```python
from build123d import *

# Parameters (mm, degrees)
BASEHEAD_DEPTH = 10
SKETCH4_W      = 0.8
SKETCH4_H      = 12.088457268


# Read off the part's stored shape, not the designer's step: HeadChamfer
with BuildPart() as part:
    # Sketch1 → BaseHead (new body)
    with BuildSketch(Plane(origin=(0, 0, 0), x_dir=(0, 0, -1), z_dir=(1, 0, 0))):
        Polygon((13.5, 7.794228634), (13.5, -7.794228634), (0, -15.588457268), (-13.5, -7.794228634), (-13.5, 7.794228634), (0, 15.588457268), align=None)
    extrude(amount=BASEHEAD_DEPTH)

    # HeadChamfer outline → HeadChamfer (revolve, cut)
    with BuildSketch(Plane.YX):
        Polygon((15.58845727, 1.205771367), (13.499999851, -8.6e-08), (15.58845727, -8.6e-08), align=None)
    revolve(axis=Axis((0, 0, 0), (1, 0, 0)), mode=Mode.SUBTRACT)

    # HeadChamfer 2 outline → HeadChamfer 2 (revolve)
    with BuildSketch(Plane.YX):
        Polygon((8, 10), (8, 108.8985), (6.8985, 110), (0, 110), (0, 10), align=None)
    revolve(axis=Axis((0, 0, 0), (1, 0, 0)))

    # Sketch4 → BearingFace (revolve, cut)
    with BuildSketch(Plane.XY, mode=Mode.PRIVATE) as bearingface_sk:
        with Locations((9.6, 19.544228634)):
            Rectangle(SKETCH4_W, SKETCH4_H)
    revolve(bearingface_sk.sketch.rotate(Axis((0, 0, 0), (1, 0, 0)), 90), axis=Axis((0, 0, 0), (1, 0, 0)), mode=Mode.SUBTRACT)


solid = part.part
```
Design review of the part built by this model. Coordinates are the model's own, in mm. A direction names the side the tool comes from. Give positions to 0.01 mm unless a question says otherwise; leave off trailing zeros. Write each loop counter-clockwise with the first axis right and the second up, starting at its lowest first coordinate (ties: lowest second). Pieces come first, ordered by that corner, then holes.
(1) Tool access review of faces 1 (the face through (9.2, -7, -12)), 2 (the face through (10, -6, 6)), 3 (the face through (9.2, 7, -12)): name each direction out of +Z, -Z, +X, -X, +Y, -Y from which nothing blocks a thin tool from reaching the whole face with its end or side.
Checked values:
face 1: -Z, +X, -Y
face 2: +X
face 3: -Z, +X, +Y
(2) Clearance check with flat-ended pins moving along their axes: pin 1 Ø4.5 at (y, z) = (-13, 0.5) entering from +X; pin 2 Ø1.5 at (x, y) = (26.5, -3) entering from +Z; pin 3 Ø1.5 at (x, y) = (97, -8) entering from -Z; pin 4 Ø7.5 at (y, z) = (4, -9.5) entering from +X. State where each tip first meets the part, or that it passes through.
Checked values:
pin 1: stops at x = 10
pin 2: stops at z = 7.68
pin 3: stops at z = -3.38
pin 4: stops at x = 110
(3) Wall thickness on line 1 along X through (y, z) = (9, -2); line 2 along X through (y, z) = (6, -4); line 3 along Y through (x, z) = (32, -2.75): over which ranges is each line inside the solid? List them lowest first.
Checked values:
line 1: x = 0 to 10
line 2: x = 0 to 109.69
line 3: y = -7.51 to 7.51
(4) Add section A-A (x = 84.5). Give the boundary of the cut face in (y, z).
Checked values:
outline: circle Ø16 at (0, 0)
